```python
from build123d import *

# Parameters (mm, degrees)
SKETCH1_R           = 51
BOSS_EXTRUDE1_DEPTH = 6
CUT_EXTRUDE1_DEPTH  = 7
SKETCH3_R           = 4
CUT_EXTRUDE2_DEPTH  = 6


with BuildPart() as part:
    # Sketch1 → Boss-Extrude1 (new body)
    with BuildSketch(Plane(origin=(0, 0, 0), x_dir=(1, 0, 0), z_dir=(0, 1, 0))):
        Circle(SKETCH1_R)
    extrude(amount=BOSS_EXTRUDE1_DEPTH)

    # Sketch2 → Cut-Extrude1 (cut, through all)
    with BuildSketch(Plane(origin=(0, 0, 0), x_dir=(1, 0, 0), z_dir=(0, 1, 0))):
        with BuildLine():
            Line((-1.779874332, 50.968932178), (-1.69262559, 48.47045511))
            ThreePointArc((-1.69262559, 48.47045511), (-4.016198064, 48.333426871), (-6.330520323, 48.085075777))
            ThreePointArc((-6.330520323, 48.085075777), (-7.191438992, 46.963104723), (-6.069467938, 46.102186054))
            ThreePointArc((-6.069467938, 46.102186054), (0, 46.5), (6.069467938, 46.102186054))
            ThreePointArc((6.069467938, 46.102186054), (7.191438992, 46.963104723), (6.330520323, 48.085075777))
            ThreePointArc((6.330520323, 48.085075777), (4.016198064, 48.333426871), (1.69262559, 48.47045511))
            Line((1.69262559, 48.47045511), (1.779874332, 50.968932178))
            ThreePointArc((1.779874332, 50.968932178), (0, 51), (-1.779874332, 50.968932178))
        make_face()
        with BuildLine():
            Line((23.943049702, 45.030327236), (22.769370795, 42.822958254))
            ThreePointArc((22.769370795, 42.822958254), (20.688583885, 43.866074555), (18.56014647, 44.808157327))
            ThreePointArc((18.56014647, 44.808157327), (17.253583505, 44.266961227), (17.794779605, 42.960398262))
            ThreePointArc((17.794779605, 42.960398262), (23.25, 40.270181276), (28.307406449, 36.890930324))
            ThreePointArc((28.307406449, 36.890930324), (29.709521218, 37.075522235), (29.524929307, 38.477637004))
            ThreePointArc((29.524929307, 38.477637004), (27.644842986, 39.84987649), (25.701084315, 41.130332664))
            Line((25.701084315, 41.130332664), (27.025882476, 43.250452904))
            ThreePointArc((27.025882476, 43.250452904), (25.5, 44.167295593), (23.943049702, 45.030327236))
        make_face()
        with BuildLine():
            Line((43.250452904, 27.025882476), (41.130332664, 25.701084315))
            ThreePointArc((41.130332664, 25.701084315), (39.84987649, 27.644842986), (38.477637004, 29.524929307))
            ThreePointArc((38.477637004, 29.524929307), (37.075522235, 29.709521218), (36.890930324, 28.307406449))
            ThreePointArc((36.890930324, 28.307406449), (40.270181276, 23.25), (42.960398262, 17.794779605))
            ThreePointArc((42.960398262, 17.794779605), (44.266961227, 17.253583505), (44.808157327, 18.56014647))
            ThreePointArc((44.808157327, 18.56014647), (43.866074555, 20.688583885), (42.822958254, 22.769370795))
            Line((42.822958254, 22.769370795), (45.030327236, 23.943049702))
            ThreePointArc((45.030327236, 23.943049702), (44.167295593, 25.5), (43.250452904, 27.025882476))
        make_face()
        with BuildLine():
            Line((50.968932178, 1.779874332), (48.47045511, 1.69262559))
            ThreePointArc((48.47045511, 1.69262559), (48.333426871, 4.016198064), (48.085075777, 6.330520323))
            ThreePointArc((48.085075777, 6.330520323), (46.963104723, 7.191438992), (46.102186054, 6.069467938))
            ThreePointArc((46.102186054, 6.069467938), (46.5, 0), (46.102186054, -6.069467938))
            ThreePointArc((46.102186054, -6.069467938), (46.963104723, -7.191438992), (48.085075777, -6.330520323))
            ThreePointArc((48.085075777, -6.330520323), (48.333426871, -4.016198064), (48.47045511, -1.69262559))
            Line((48.47045511, -1.69262559), (50.968932178, -1.779874332))
            ThreePointArc((50.968932178, -1.779874332), (51, 0), (50.968932178, 1.779874332))
        make_face()
        with BuildLine():
            Line((45.030327236, -23.943049702), (42.822958254, -22.769370795))
            ThreePointArc((42.822958254, -22.769370795), (43.866074555, -20.688583885), (44.808157327, -18.56014647))
            ThreePointArc((44.808157327, -18.56014647), (44.266961227, -17.253583505), (42.960398262, -17.794779605))
            ThreePointArc((42.960398262, -17.794779605), (40.270181276, -23.25), (36.890930324, -28.307406449))
            ThreePointArc((36.890930324, -28.307406449), (37.075522235, -29.709521218), (38.477637004, -29.524929307))
            ThreePointArc((38.477637004, -29.524929307), (39.84987649, -27.644842986), (41.130332664, -25.701084315))
            Line((41.130332664, -25.701084315), (43.250452904, -27.025882476))
            ThreePointArc((43.250452904, -27.025882476), (44.167295593, -25.5), (45.030327236, -23.943049702))
        make_face()
        with BuildLine():
            Line((27.025882476, -43.250452904), (25.701084315, -41.130332664))
            ThreePointArc((25.701084315, -41.130332664), (27.644842986, -39.84987649), (29.524929307, -38.477637004))
            ThreePointArc((29.524929307, -38.477637004), (29.709521218, -37.075522235), (28.307406449, -36.890930324))
            ThreePointArc((28.307406449, -36.890930324), (23.25, -40.270181276), (17.794779605, -42.960398262))
            ThreePointArc((17.794779605, -42.960398262), (17.253583505, -44.266961227), (18.56014647, -44.808157327))
            ThreePointArc((18.56014647, -44.808157327), (20.688583885, -43.866074555), (22.769370795, -42.822958254))
            Line((22.769370795, -42.822958254), (23.943049702, -45.030327236))
            ThreePointArc((23.943049702, -45.030327236), (25.5, -44.167295593), (27.025882476, -43.250452904))
        make_face()
        with BuildLine():
            Line((1.779874332, -50.968932178), (1.69262559, -48.47045511))
            ThreePointArc((1.69262559, -48.47045511), (4.016198064, -48.333426871), (6.330520323, -48.085075777))
            ThreePointArc((6.330520323, -48.085075777), (7.191438992, -46.963104723), (6.069467938, -46.102186054))
            ThreePointArc((6.069467938, -46.102186054), (0, -46.5), (-6.069467938, -46.102186054))
            ThreePointArc((-6.069467938, -46.102186054), (-7.191438992, -46.963104723), (-6.330520323, -48.085075777))
            ThreePointArc((-6.330520323, -48.085075777), (-4.016198064, -48.333426871), (-1.69262559, -48.47045511))
            Line((-1.69262559, -48.47045511), (-1.779874332, -50.968932178))
            ThreePointArc((-1.779874332, -50.968932178), (0, -51), (1.779874332, -50.968932178))
        make_face()
        with BuildLine():
            Line((-23.943049702, -45.030327236), (-22.769370795, -42.822958254))
            ThreePointArc((-22.769370795, -42.822958254), (-20.688583885, -43.866074555), (-18.56014647, -44.808157327))
            ThreePointArc((-18.56014647, -44.808157327), (-17.253583505, -44.266961227), (-17.794779605, -42.960398262))
            ThreePointArc((-17.794779605, -42.960398262), (-23.25, -40.270181276), (-28.307406449, -36.890930324))
            ThreePointArc((-28.307406449, -36.890930324), (-29.709521218, -37.075522235), (-29.524929307, -38.477637004))
            ThreePointArc((-29.524929307, -38.477637004), (-27.644842986, -39.84987649), (-25.701084315, -41.130332664))
            Line((-25.701084315, -41.130332664), (-27.025882476, -43.250452904))
            ThreePointArc((-27.025882476, -43.250452904), (-25.5, -44.167295593), (-23.943049702, -45.030327236))
        make_face()
        with BuildLine():
            Line((-43.250452904, -27.025882476), (-41.130332664, -25.701084315))
            ThreePointArc((-41.130332664, -25.701084315), (-39.84987649, -27.644842986), (-38.477637004, -29.524929307))
            ThreePointArc((-38.477637004, -29.524929307), (-37.075522235, -29.709521218), (-36.890930324, -28.307406449))
            ThreePointArc((-36.890930324, -28.307406449), (-40.270181276, -23.25), (-42.960398262, -17.794779605))
            ThreePointArc((-42.960398262, -17.794779605), (-44.266961227, -17.253583505), (-44.808157327, -18.56014647))
            ThreePointArc((-44.808157327, -18.56014647), (-43.866074555, -20.688583885), (-42.822958254, -22.769370795))
            Line((-42.822958254, -22.769370795), (-45.030327236, -23.943049702))
            ThreePointArc((-45.030327236, -23.943049702), (-44.167295593, -25.5), (-43.250452904, -27.025882476))
        make_face()
        with BuildLine():
            Line((-50.968932178, -1.779874332), (-48.47045511, -1.69262559))
            ThreePointArc((-48.47045511, -1.69262559), (-48.333426871, -4.016198064), (-48.085075777, -6.330520323))
            ThreePointArc((-48.085075777, -6.330520323), (-46.963104723, -7.191438992), (-46.102186054, -6.069467938))
            ThreePointArc((-46.102186054, -6.069467938), (-46.5, 0), (-46.102186054, 6.069467938))
            ThreePointArc((-46.102186054, 6.069467938), (-46.963104723, 7.191438992), (-48.085075777, 6.330520323))
            ThreePointArc((-48.085075777, 6.330520323), (-48.333426871, 4.016198064), (-48.47045511, 1.69262559))
            Line((-48.47045511, 1.69262559), (-50.968932178, 1.779874332))
            ThreePointArc((-50.968932178, 1.779874332), (-51, 0), (-50.968932178, -1.779874332))
        make_face()
        with BuildLine():
            Line((-45.030327236, 23.943049702), (-42.822958254, 22.769370795))
            ThreePointArc((-42.822958254, 22.769370795), (-43.866074555, 20.688583885), (-44.808157327, 18.56014647))
            ThreePointArc((-44.808157327, 18.56014647), (-44.266961227, 17.253583505), (-42.960398262, 17.794779605))
            ThreePointArc((-42.960398262, 17.794779605), (-40.270181276, 23.25), (-36.890930324, 28.307406449))
            ThreePointArc((-36.890930324, 28.307406449), (-37.075522235, 29.709521218), (-38.477637004, 29.524929307))
            ThreePointArc((-38.477637004, 29.524929307), (-39.84987649, 27.644842986), (-41.130332664, 25.701084315))
            Line((-41.130332664, 25.701084315), (-43.250452904, 27.025882476))
            ThreePointArc((-43.250452904, 27.025882476), (-44.167295593, 25.5), (-45.030327236, 23.943049702))
        make_face()
        with BuildLine():
            Line((-27.025882476, 43.250452904), (-25.701084315, 41.130332664))
            ThreePointArc((-25.701084315, 41.130332664), (-27.644842986, 39.84987649), (-29.524929307, 38.477637004))
            ThreePointArc((-29.524929307, 38.477637004), (-29.709521218, 37.075522235), (-28.307406449, 36.890930324))
            ThreePointArc((-28.307406449, 36.890930324), (-23.25, 40.270181276), (-17.794779605, 42.960398262))
            ThreePointArc((-17.794779605, 42.960398262), (-17.253583505, 44.266961227), (-18.56014647, 44.808157327))
            ThreePointArc((-18.56014647, 44.808157327), (-20.688583885, 43.866074555), (-22.769370795, 42.822958254))
            Line((-22.769370795, 42.822958254), (-23.943049702, 45.030327236))
            ThreePointArc((-23.943049702, 45.030327236), (-25.5, 44.167295593), (-27.025882476, 43.250452904))
        make_face()
    extrude(amount=CUT_EXTRUDE1_DEPTH, mode=Mode.SUBTRACT)

    # Sketch3 → Cut-Extrude2 (cut)
    with BuildSketch(Plane(origin=(0, 0, 0), x_dir=(1, 0, 0), z_dir=(0, 1, 0))):
        Circle(SKETCH3_R)
    extrude(amount=CUT_EXTRUDE2_DEPTH, mode=Mode.SUBTRACT)


solid = part.part
```
CAD build for the part. Positions are in the model's coordinates, mm. A direction names the side the tool comes from. Round coordinates to 2 decimals unless told otherwise and drop trailing zeros. Order: outer loops, then holes, each group sorted by start corner. A loop starts at its lowest first (then second) coordinate and runs counter-clockwise, first axis right, second up.
Item 1: Mould opens along X. For faces 3 (the face through (-27.67, 2.96, 39.83)), 4 (the face through (11, 6, -1)), 5 (the face through (-13.043, 2.958, -49.304)) say: pulls with the +X half, pulls with the -X half, needs draft (parallel to the pull), parting line crosses it, or undercut.
Item 2: Tool access for faces 1 (the face through (-27.618, 2.958, -39.868)), 2 (the face through (11, 0, -1)): list every direction of +Z, -Z, +X, -X, +Y, -Y with a clear straight run to the whole face (end or side of a thin tool).
Item 3: Saw through at D-D on z = -13. Write the cut outline in (x, y), then the cut area to 3 significant figures.
Item 4: Saw through at B-B on z = 0. Write the cut outline in (x, y).
Item 5: Saw through at C-C on x = -20. Write the cut outline in (y, z).
Item 6: Pin check, flat tips, straight feed: pin 1 (1 mm diameter, centred on y = 3, z = -9, fed in from -X); pin 2 (2 mm diameter, centred on x = -16, z = -29, fed in from -Y); pin 3 (1 mm diameter, centred on x = -35, y = 1, fed in from +Z); pin 4 (1.5 mm diameter, centred on y = 3, z = 40, fed in from +X). Stop position of each tip, or through.
Item 7: Probe line 1 along X through (y, z) = (1.95, 0); line 2 along X through (y, z) = (2.75, 27). List the from-to ranges inside material, lowest first.
Item 8: Saw through at A-A on x = 0. Write the cut outline in (y, z).
Reported:
1. face 3: undercut
1. face 4: needs draft
1. face 5: pulls with the -X half
2. face 1: +Y, -Y
2. face 2: +Z, -Z, +X, -X, -Y
3. outline: (-49.32, 0) - (49.32, 0) - (49.32, 6) - (-49.32, 6) - close
3. area: 592 mm2
4. outline: (-46.5, 0) - (-4, 0) - (-4, 6) - (-46.5, 6) - close; (4, 0) - (46.5, 0) - (46.5, 6) - (4, 6) - close
5. outline: (0, -46.91) - (6, -46.91) - (6, -44.18) - (0, -44.18) - close; (0, -41.98) - (6, -41.98) - (6, 41.98) - (0, 41.98) - close; (0, 44.18) - (6, 44.18) - (6, 46.91) - (0, 46.91) - close
6. pin 1: stops at x = -50.29
6. pin 2: stops at y = 0
6. pin 3: stops at z = 37.56
6. pin 4: stops at x = 32.56
7. line 1: x = -46.5 to -4, 4 to 46.5
7. line 2: x = -43.21 to -40.29, -37.86 to 37.86, 40.29 to 43.21
8. outline: (0, -46.5) - (6, -46.5) - (6, -4) - (0, -4) - close; (0, 4) - (6, 4) - (6, 46.5) - (0, 46.5) - close
